For this review, use the dimensioned drawing (mm, ordinates from the lowest corner) and the shaded views. A direction names the side the tool comes from. Round coordinates to 2 decimals unless told otherwise and drop trailing zeros. Write each loop counter-clockwise with the first axis right and the second up, starting at its lowest first coordinate (ties: lowest second). Pieces come first, ordered by that corner, then holes.
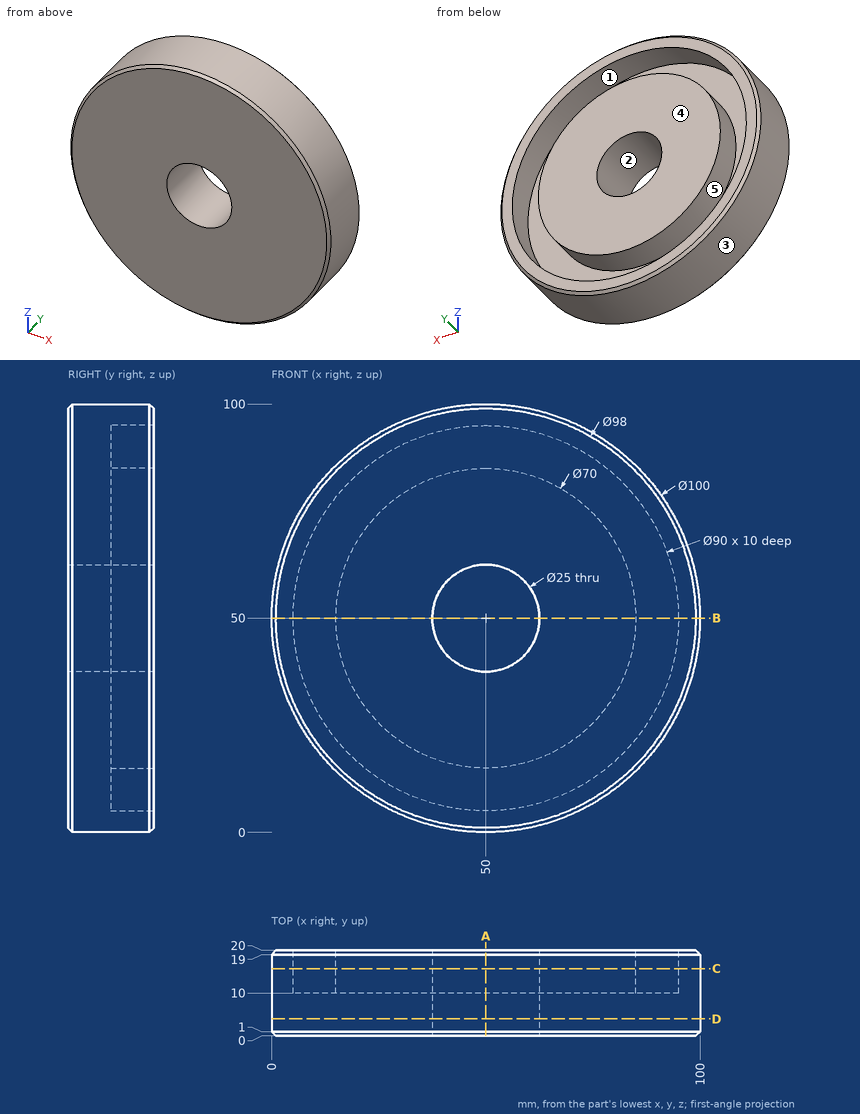
1) Add section A-A on x = 50. State the section outline as (y, z) points.
2) For the marked faces 1 and 2, list the 3-axis set-ups (+Z, -Z, +X, -X, +Y, -Y) from which the entire face can be reached by the end or side of a thin tool; tool diameter is ignored.
3) Add section B-B on z = 50. State the section outline as (x, y) points, and give its area (3 significant figures).
4) Add section D-D on y = 4. State the section outline as (x, z) points, and give its area (3 significant figures).
5) The part is to be moulded in two halves that separate along X. For the marked faces 3, 4 and 5, say which applies: pulls with the +X half, pulls with the -X half, needs draft (parallel to the pull), parting line crosses it, or undercut.
6) For P1, Ø8, axis at y = 10.5, z = 46, coming from the -X side; P2, Ø2, axis at x = 59.5, y = 6, coming from the +Z side; P3, Ø12, axis at x = 74, y = 17, coming from the -Z side, all flat-tipped, find the tip position at first contact; note any pin that passes through.
7) Add section C-C on y = 15.75. State the section outline as (x, z) points.
8) For line 1 along X through (y, z) = (16, 50); line 2 along X through (y, z) = (6.25, 50); line 3 along Z through (x, y) = (47, 17.25), list the stretches that pass through material, from the lowest coordinate up.
Computed:
1. outline: (0, 1) - (1, 0) - (19, 0) - (20, 1) - (20, 5) - (10, 5) - (10, 15) - (20, 15) - (20, 37.5) - (0, 37.5) - close; (0, 62.5) - (20, 62.5) - (20, 85) - (10, 85) - (10, 95) - (20, 95) - (20, 99) - (19, 100) - (1, 100) - (0, 99) - close
2. face 1: +Y
2. face 2: +Y, -Y
3. outline: (0, 1) - (1, 0) - (37.5, 0) - (37.5, 20) - (15, 20) - (15, 10) - (5, 10) - (5, 20) - (1, 20) - (0, 19) - close; (62.5, 0) - (99, 0) - (100, 1) - (100, 19) - (99, 20) - (95, 20) - (95, 10) - (85, 10) - (85, 20) - (62.5, 20) - close
3. area: 1,300 mm2
4. outline: circle Ø100 at (50, 50); hole circle Ø25 at (50, 50)
4. area: 7,360 mm2
5. face 3: parting line crosses it
5. face 4: needs draft
5. face 5: undercut
6. P1: stops at x = 0
6. P2: stops at z = 99.27
6. P3: stops at z = 3.35
7. outline: circle Ø100 at (50, 50); circle Ø70 at (50, 50); hole circle Ø90 at (50, 50); hole circle Ø25 at (50, 50)
8. line 1: x = 0 to 5, 15 to 37.5, 62.5 to 85, 95 to 100
8. line 2: x = 0 to 37.5, 62.5 to 100
8. line 3: z = 0.09 to 5.1, 15.13 to 37.87, 62.13 to 84.87, 94.9 to 99.91
